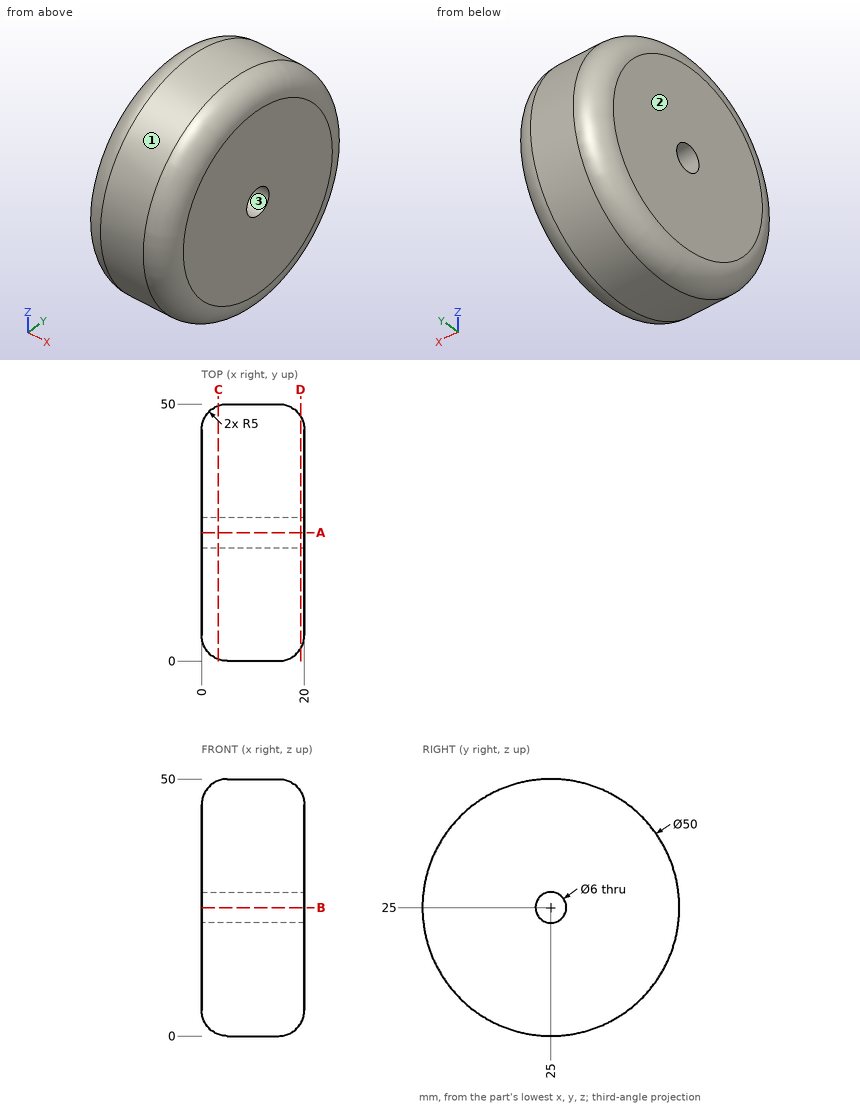
For this review, use the dimensioned drawing (mm, ordinates from the lowest corner) and the shaded views. Round coordinates to 2 decimals unless told otherwise and drop trailing zeros. Loops run counter-clockwise (first coordinate to the right, second up) from the corner with the lowest first, then second, coordinate; pieces in that order, holes last. Notation, with made-up numbers: M 5.25,45 L 39.25,45 A22 cw 39.25,82 Z; hole C 39,36.25 d5. An arc over 180 degrees is marked long. Answer as a JSON object with one key per item and string values.
(1) Draft analysis for pull direction Z (two halves, no side actions). For the marked faces 1, 2 and 3, state which applies: released by +Z, released by -Z, zero draft, split by the parting line, or undercut.
Resolved:
{"face 1": "split by the parting line", "face 2": "zero draft", "face 3": "undercut"}
(2) Take a section at D-D on x = 19.25. Give the boundary of the cut face in (y, z), and give its area (3 significant figures).
Resolved:
{"outline": "C 25,25 d45.27; hole C 25,25 d6", "area": "1,580 mm²"}
(3) Take a section at C-C on x = 3.25. Give the boundary of the cut face in (y, z).
Resolved:
{"outline": "C 25,25 d49.37; hole C 25,25 d6"}
(4) Take a section at A-A on y = 25. Give the boundary of the cut face in (x, z), and give its area (3 significant figures).
Resolved:
{"outline": "M 0,5 A5 ccw 5,0 L 15,0 A5 ccw 20,5 L 20,22 L 0,22 Z; M 0,28 L 20,28 L 20,45 A5 ccw 15,50 L 5,50 A5 ccw 0,45 Z", "area": "859 mm²"}
(5) To check wall thickness, follow line 1 along Y through (x, z) = (4.75, 10); line 2 along Z through (x, y) = (10.5, 26); line 3 along Z through (x, y) = (8.5, 23). State the ranges of each line that lie inside material, in increasing order.
Resolved:
{"line 1": "5.01 to 44.99", "line 2": "0.02 to 22.17, 27.83 to 49.98", "line 3": "0.08 to 22.76, 27.24 to 49.92"}
(6) Clearance check with flat-ended pins moving along their axes: P1, Ø3, axis at x = 2.5, y = 12, coming from the +Z side; P2, Ø5, axis at x = 16, y = 7.5, coming from the +Z side; P3, Ø1.5, axis at x = 5.5, z = 22.5, coming from the +Y side. State where each tip first meets the part, or that it passes through.
Resolved:
{"P1": "z = 46.74", "P2": "z = 44.93", "P3": "y = 49.94"}
